Geometry: final body of the model. Coordinates: model frame, mm. Give positions to 0.01 mm unless a question says otherwise; leave off trailing zeros. Loops run counter-clockwise (first coordinate to the right, second up) from the corner with the lowest first, then second, coordinate; pieces in that order, holes last. Notation, with made-up numbers: (48.5, 6) -> (100.5, 6) arc R26 ccw to (100.5, 45) -> close; hole circle Ø9 at (72.25, 48). An arc over 180 degrees is marked (long way). Answer in a Markdown table with one row per item. Add a question column.
1) Line query: line 1 (Y direction, x = 16.5, z = 2); line 2 (Y direction, x = 21, z = 3.5); line 3 (Y direction, x = 54, z = 3). Output: solid intervals per line, ascending. Write a range as from..to.
2) First-contact query: P1, Ø6.5, axis at x = 57.15, y = 57.15, coming from the +Z side. Flat tip, straight axial feed; report the tip coordinate or a pass-through.
3) Section query C-C (x = 47). Return the cut outline in (y, z), plus the area to 3 significant figures.
4) Section query B-B (z = 3). Give the number of separate pieces and of enclosed holes in the cut face, plus the area to 3 significant figures.
5) Draft query along Y for faces 1 (the flat face through (76.2, 132, 3)), 2 (the cylindrical face through (58.05, 243.95, 3.13)), 3 (the flat face through (67.41, 274.82, 3.13)). Return one class per face: +Y half, -Y half, draft (parallel to the pull), parting line (faces both ways), or undercut.
6) Section query A-A (y = 19.05). Return the cut outline in (x, z).
```python
from build123d import *

# Parameters (mm, degrees)
BOSS_EXTRUDE1_DEPTH              = 6.35
F_21_64_0_32813_DIAMETER_HOLE1_D = 8.334502
LPATTERN1_COUNT                  = 2
LPATTERN1_PITCH                  = 38.1
LPATTERN1_COUNT_DIR2             = 2
LPATTERN1_PITCH_DIR2             = 38.1
F_21_64_0_32813_DIAMETER_HOLE2_D = 8.334502
LPATTERN2_COUNT                  = 3
LPATTERN2_PITCH                  = 57.15
LPATTERN2_COUNT_DIR2             = 2
LPATTERN2_PITCH_DIR2             = 38.1


with BuildPart() as part:
    # Sketch2 → Boss-Extrude1 (new body)
    with BuildSketch(Plane.XY):
        Polygon((0, 0), (76.2, 0), (76.2, 268.269814476), (58.378218394, 281.548923082), (0, 203.2), align=None)
    extrude(amount=BOSS_EXTRUDE1_DEPTH)

    # 21/64 (0.32813) Diameter Hole1 (through all)
    with Locations(Plane.XY.offset(6.35)):
        with Locations((57.15, 19.05)):
            f_21_64_0_32813_diameter_hole1 = Hole(F_21_64_0_32813_DIAMETER_HOLE1_D / 2)

    # LPattern1: 21_64 _0.32813_ Diameter Hole1 2 × 2
    with Locations(*[(-i * LPATTERN1_PITCH, j * LPATTERN1_PITCH_DIR2, 0) for i in range(LPATTERN1_COUNT) for j in range(LPATTERN1_COUNT_DIR2) if (i, j) != (0, 0)]):
        add(f_21_64_0_32813_diameter_hole1, mode=Mode.SUBTRACT)

    # 21/64 (0.32813) Diameter Hole2 (through all)
    with Locations(Plane.XY.offset(6.35)):
        with Locations((57.15, 248.0169065)):
            f_21_64_0_32813_diameter_hole2 = Hole(F_21_64_0_32813_DIAMETER_HOLE2_D / 2)

    # LPattern2: 21_64 _0.32813_ Diameter Hole2 3 × 2, 2 skipped
    with Locations(*[Vector(-0.5974852016253348, -0.8018799372965589, 0) * (i * LPATTERN2_PITCH) + Vector(0.8018799372965594, -0.5974852016253339, 0) * (j * LPATTERN2_PITCH_DIR2) for i in range(LPATTERN2_COUNT) for j in range(LPATTERN2_COUNT_DIR2) if (i, j) not in ((0, 0), (0, 1), (2, 0))]):
        add(f_21_64_0_32813_diameter_hole2, mode=Mode.SUBTRACT)


solid = part.part
```
Evaluation:
| question | item | result |
|---|---|---|
| 1 | line 1 | 0..15.75, 22.35..53.85, 60.45..130.61, 136.58..225.34 |
| 1 | line 2 | 0..15.37, 22.73..53.47, 60.83..129.75, 137.45..198.54, 205.84..231.38 |
| 1 | line 3 | 0..16.32, 21.78..54.42, 59.88..175.28, 183.57..245.29, 250.75..275.67 |
| 2 | P1 | through |
| 3 | outline | (0, 0) -> (266.28, 0) -> (266.28, 6.35) -> (0, 6.35) -> close |
| 3 | area | 1,690 mm² |
| 4 | separate pieces | 1 |
| 4 | enclosed holes | 8 |
| 4 | area | 18,600 mm² |
| 5 | face 1 | draft |
| 5 | face 2 | undercut |
| 5 | face 3 | +Y half |
| 6 | outline | (0, 0) -> (14.88, 0) -> (14.88, 6.35) -> (0, 6.35) -> close; (23.22, 0) -> (52.98, 0) -> (52.98, 6.35) -> (23.22, 6.35) -> close; (61.32, 0) -> (76.2, 0) -> (76.2, 6.35) -> (61.32, 6.35) -> close |
